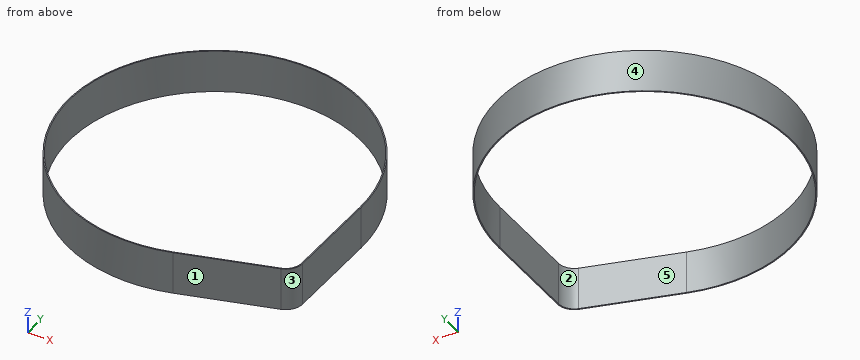
Autodesk Inventor part; units mm, degrees
ref_plane "YZ Plane" through (0, 0, 0) normal (1, 0, 0) x (0, 1, 0)
ref_plane "XZ Plane" through (0, 0, 0) normal (0, 1, 0) x (-1, 0, 0)
ref_plane "XY Plane" through (0, 0, 0) normal (0, 0, 1) x (1, 0, 0)
sketch "Sketch1" plane through (0, 0, 0) normal (0, 0, 1) x (1, 0, 0)
  circle A0 centre (0, 0) radius 101.6 construction
  arc A1 (78.464, -64.852) -> (82.3203, -59.5483) centre (88.8846, -68.3749) ccw construction
  line L0 (101.5669, -2.5919) -> (99.881, -68.6555)
  line L1 (91.9762, -78.9315) -> (28.5548, -97.5048)
  arc A2 (101.5669, -2.5919) -> (28.5548, -97.5048) centre (0, 0) ccw
  arc A3 (91.9762, -78.9315) -> (99.881, -68.6555) centre (88.8846, -68.3749) ccw
  line L2 (100.6577, -68.6753) -> (102.3436, -2.6117)
  arc A4 (102.3436, -2.6117) -> (28.7731, -98.2504) centre (0, 0) ccw
  line L3 (28.7731, -98.2504) -> (92.1945, -79.6771)
  arc A5 (92.1945, -79.6771) -> (100.6577, -68.6753) centre (88.8846, -68.3749) ccw
  point P0 (0, 0)
  dimension "d0" = 0.7769
extrude "Extrusion1" add sketch "Sketch1" against normal blind 30
properties part number "PoleHeightMarker"
Read the model definition and answer for the solid it produces. Units are mm, in the model's axes. Face numbers are marked on the shaded views. A direction names the side the tool comes from. Coordinates: 2 decimals unless noted, no trailing zeros. Write each loop counter-clockwise with the first axis right and the second up, starting at its lowest first coordinate (ties: lowest second). Pieces come first, ordered by that corner, then holes. Notation, with made-up numbers: (36, 40.25) - (58, 40.25) arc R19 cw to (58, 49.25) - close; hole circle Ø8 at (86, 27). An arc over 180 degrees is marked (long way). Answer as a JSON object with one key per item and string values. Group by question number.
1. A cutting plane is placed at C-C (x = 85.5). Determine the outline of the cut face in (y, z).
2. A cutting plane is placed at B-B (y = -18). Determine the outline of the cut face in (x, z).
3. A cutting plane is placed at A-A (z = -10). Determine the outline of the cut face in (x, y).
4. The mould has two halves that part along X. Classify the marked faces 3, 4 and 5: +X half, -X half, draft (parallel to the pull), parting line (faces both ways), or undercut.
5. Each of these flat-tipped pins is pushed along its axis until it touches: P1, Ø5, axis at y = -5.5, z = -20, coming from the -X side; P2, Ø10, axis at y = 59.5, z = -10.5, coming from the +X side; P3, Ø1.5, axis at y = 44, z = -25.5, coming from the +X side. Where does it stop, or does it pass through?
6. Consider L1, parallel to X at y = 1, z = -26.25; L2, parallel to X at y = 15, z = -25.75; L3, parallel to Y at x = 75, z = -28. Determine where each line is inside the solid, lowest interval first. Write a range as [from, to].
7. Which of the six approach directions +Z, -Z, +X, -X, +Y, -Y give full straight-line access (tool end or side, diameter ignored) to the marked faces 1 and 2?
Worked out:
{
 "1": {"outline": "(-81.64, -30) - (-80.83, -30) - (-80.83, 0) - (-81.64, 0) - close; (54.88, -30) - (56.31, -30) - (56.31, 0) - (54.88, 0) - close"},
 "2": {"outline": "(-100.78, -30) - (-99.99, -30) - (-99.99, 0) - (-100.78, 0) - close; (101.17, -30) - (101.95, -30) - (101.95, 0) - (101.17, 0) - close"},
 "3": {"outline": "(28.77, -98.25) - (92.19, -79.68) arc R11.78 ccw to (100.66, -68.68) - (102.34, -2.61) arc R102.38 ccw (long way) to start; hole (28.55, -97.5) - (91.98, -78.93) arc R11 ccw to (99.88, -68.66) - (101.57, -2.59) arc R101.6 ccw (long way) to start"},
 "4": {"face 3": "+X half", "face 4": "parting line", "face 5": "undercut"},
 "5": {"P1": "stops at x = -102.33", "P2": "stops at x = 86.66", "P3": "stops at x = 92.79"},
 "6": {"L1": "x = [-102.37, -101.6], [101.6, 102.37]", "L2": "x = [-101.27, -100.49], [100.49, 101.27]", "L3": "y = [-84.71, -83.9], [68.54, 69.69]"},
 "7": {"face 1": "+Z, -Z, +X, -Y", "face 2": "+Z, -Z"}
}
